Check sheet for the modelled part. Datum: model origin and axes. Units: mm. Face numbers are marked on the shaded views. A direction names the side the tool comes from. Give positions to 0.01 mm unless a question says otherwise; leave off trailing zeros. Write each loop counter-clockwise with the first axis right and the second up, starting at its lowest first coordinate (ties: lowest second). Pieces come first, ordered by that corner, then holes. Notation, with made-up numbers: M -13.5,23.5 L 26.5,23.5 A12 cw 26.5,29.5 Z; hole C 1,-27 d3. An arc over 180 degrees is marked long. Use CSV: the item, a comma, the result in double quotes. Start each with the question number.
1. Cross-section at D-D, the plane y = 15.5. Enter the section's corners in (x, z).
2. Cross-section at C-C, the plane z = 9. Enter the section's corners in (x, y).
3. Scan lines: line 1 (Y direction, x = 0, z = 4.5); line 2 (X direction, y = 0.5, z = 5); line 3 (Y direction, x = 0, z = 7.65). Record each from-to range of solid material in increasing order.
4. Access from +Z, -Z, +X, -X, +Y, -Y to the whole of each face (thin tool, end or side, straight path). Record for the marked faces 5 and 6.
5. Cross-section at A-A, the plane x = 0. Enter the section's corners in (y, z), and give its area (3 significant figures).
6. Depth check by flat-ended pin: P1, Ø5, axis at y = -17, z = 4.5, coming from the -X side; P2, Ø23, axis at x = 6.5, y = -4.5, coming from the +Z side; P3, Ø4, axis at y = -23, z = 9, coming from the -X side; P4, Ø4, axis at x = -9, y = -3, coming from the -Z side. Enter the tip coordinate at first touch or a pass-through.
7. Cross-section at B-B, the plane z = 2.5. Enter the section's corners in (x, y).
8. Mould release check, pull along X, two halves, no side actions. Record for the marked faces 1, 2, 3 and 4: +X half, -X half, draft (parallel to the pull), parting line (faces both ways), or undercut.
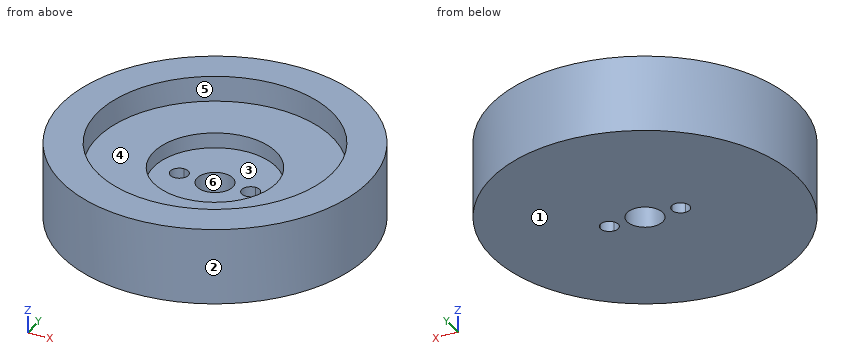
from build123d import *

# Parameters (mm, degrees)
F0_R     = 30
F1_DEPTH = 15
F3_DEPTH = 25
F4_R     = 23
F5_DEPTH = 5
F6_R     = 12
F7_DEPTH = 3
F8_R     = 3.5
F9_DEPTH = 25


with BuildPart() as f1:
    # F0 (on Top) → F1 (new body)
    with BuildSketch(Plane.XY):
        Circle(F0_R)
    extrude(amount=F1_DEPTH)

    # F2 (on face) → F3 (cut)
    with BuildSketch(Plane.XY.offset(15)):
        with BuildLine():
            ThreePointArc((-5.25, 0), (-5.7625631329, 1.2374368671), (-7, 1.75))
            Line((-7, 1.75), (-7, -1.75))
            ThreePointArc((-7, -1.75), (-5.7625631329, -1.2374368671), (-5.25, 0))
        make_face()
        with BuildLine():
            Line((-7, -1.75), (-7, 1.75))
            ThreePointArc((-7, 1.75), (-8.75, 0), (-7, -1.75))
        make_face()
        with BuildLine():
            Line((7, -1.75), (7, 1.75))
            ThreePointArc((7, 1.75), (5.25, 0), (7, -1.75))
        make_face()
        with BuildLine():
            ThreePointArc((8.75, 0), (8.2374368671, 1.2374368671), (7, 1.75))
            Line((7, 1.75), (7, -1.75))
            ThreePointArc((7, -1.75), (8.2374368671, -1.2374368671), (8.75, 0))
        make_face()
    extrude(amount=-F3_DEPTH, mode=Mode.SUBTRACT)

    # F4 (on face) → F5 (cut)
    with BuildSketch(Plane.XY.offset(15)):
        Circle(F4_R)
    extrude(amount=-F5_DEPTH, mode=Mode.SUBTRACT)

    # F6 (on face) → F7 (cut)
    with BuildSketch(Plane.XY.offset(10)):
        Circle(F6_R)
    extrude(amount=-F7_DEPTH, mode=Mode.SUBTRACT)

    # F8 (on face) → F9 (cut)
    with BuildSketch(Plane(origin=(0, 0, 0), x_dir=(1, 0, 0), z_dir=(0, 0, -1))):
        Circle(F8_R)
    extrude(amount=-F9_DEPTH, mode=Mode.SUBTRACT)


solid = f1.part
Worked answers:
1,outline,"M -25.69,0 L 25.69,0 L 25.69,15 L 16.99,15 L 16.99,10 L -16.99,10 L -16.99,15 L -25.69,15 Z"
2,outline,"C 0,0 d60; hole C 0,0 d24"
3,line 1,"y = -30 to -3.5, 3.5 to 30"
3,line 2,"x = -30 to -8.68, -5.32 to -3.46, 3.46 to 5.32, 8.68 to 30"
3,line 3,"y = -30 to -12, 12 to 30"
4,face 5,"+Z"
4,face 6,"+Z, -Z"
5,outline,"M -30,0 L -3.5,0 L -3.5,7 L -12,7 L -12,10 L -23,10 L -23,15 L -30,15 Z; M 3.5,0 L 30,0 L 30,15 L 23,15 L 23,10 L 12,10 L 12,7 L 3.5,7 Z"
5,area,"549 mm^2"
6,P1,"stops at x = -26.26"
6,P2,"stops at z = 10"
6,P3,"stops at x = -21.42"
6,P4,"stops at z = 0"
7,outline,"C 0,0 d60; hole C -7,0 d3.5; hole C 0,0 d7; hole C 7,0 d3.5"
8,face 1,"draft"
8,face 2,"parting line"
8,face 3,"undercut"
8,face 4,"undercut"
